```python
from build123d import *

# Parameters (mm, degrees)
CROQUIS1_R              = 2.5
SALIENTE_EXTRUIR1_DEPTH = 6
CROQUIS4_R              = 1
CORTAR_EXTRUIR2_DEPTH   = 3.2


with BuildPart() as part:
    # Croquis1 → Saliente-Extruir1 (new body)
    with BuildSketch(Plane.XY):
        with BuildLine():
            Line((-3.15, -10), (-3.15, -3.545259156))
            Line((-3.15, -3.545259156), (-4, 0))
            ThreePointArc((-4, 0), (0, 4), (4, 0))
            ThreePointArc((4, 0), (2.759247212, -2.590701364), (0.05, -3.545259156))
            Line((0.05, -3.545259156), (0.05, -10))
            Line((0.05, -10), (-3.15, -10))
        make_face()
        Circle(CROQUIS1_R, mode=Mode.SUBTRACT)
    extrude(amount=SALIENTE_EXTRUIR1_DEPTH)

    # Croquis4 → Cortar-Extruir2 (cut)
    with BuildSketch(Plane(origin=(0.05, 0, 0), x_dir=(0, 0, -1), z_dir=(1, 0, 0))):
        with Locations((-3, -6.050719138)):
            Circle(CROQUIS4_R)
    extrude(amount=-CORTAR_EXTRUIR2_DEPTH, mode=Mode.SUBTRACT)


solid = part.part
```
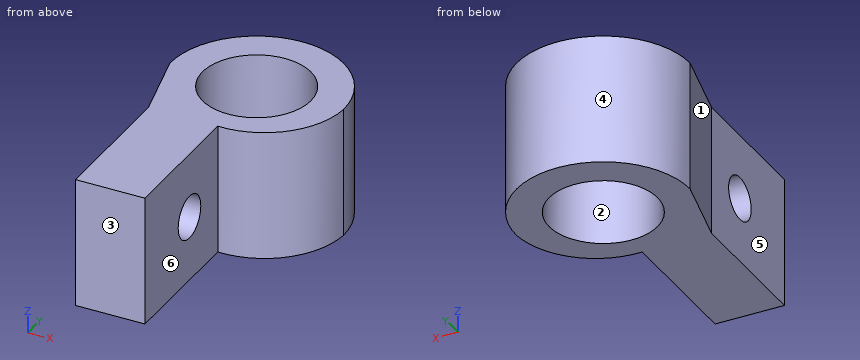
Can you work these out from the model? Positions are in its coordinate system, mm. Face numbers are marked on the shaded views. A direction names the side the tool comes from. Coordinates: 2 decimals unless noted, no trailing zeros. Order: outer loops, then holes, each group sorted by start corner. A loop starts at its lowest first (then second) coordinate and runs counter-clockwise, first axis right, second up. Notation, with made-up numbers: (31.5, 29.25) - (42.5, 29.25) arc R17 ccw to (42.5, 60.25) - close; hole circle Ø5 at (-36, 24.25). An arc over 180 degrees is marked (long way). Answer in a Markdown table with one row per item.
1. For pin 1 (1.5 mm diameter, centred on x = -1, y = -3, fed in from -Z); pin 2 (2 mm diameter, centred on x = -3, z = 1, fed in from +Y); pin 3 (2.5 mm diameter, centred on y = -6.05, z = 3, fed in from +X), each with a flat end and sliding along its axis, tell me the tip position at first contact or that it passes through.
Reply:
| item | result |
|---|---|
| pin 1 | stops at z = 0 |
| pin 2 | stops at y = 3.46 |
| pin 3 | stops at x = 0.05 |
2. Suppose I cut it at D-D (x = 2.25). Please give me the cut outline in (y, z), and give its area (3 significant figures).
Reply:
| item | result |
|---|---|
| outline | (-2.97, 0) - (-1.09, 0) - (-1.09, 6) - (-2.97, 6) - close; (1.09, 0) - (3.31, 0) - (3.31, 6) - (1.09, 6) - close |
| area | 24.6 mm^2 |
3. For the marked faces 4, 5 and 6, which set-ups out of +Z, -Z, +X, -X, +Y, -Y let a thin tool reach every point of the face, with its end or its side?
Reply:
| item | result |
|---|---|
| face 4 | +Z, -Z, +Y |
| face 5 | +Z, -Z, -X, -Y |
| face 6 | +Z, -Z, +X, -Y |
4. If I drill on line 1 along Y through (x, z) = (0, 1.5); line 2 along X through (y, z) = (-6.75, 4.5); line 3 along Y through (x, z) = (-1.4, 3), over which ranges is the centre line in solid material (lowest first)?
Reply:
| item | result |
|---|---|
| line 1 | y = -10 to -2.5, 2.5 to 4 |
| line 2 | x = -3.15 to 0.05 |
| line 3 | y = -10 to -7.05, -5.05 to -2.07, 2.07 to 3.75 |
5. Suppose I cut it at A-A (z = 3). Please give me the cut outline in (x, y), and give its area (3 significant figures).
Reply:
| item | result |
|---|---|
| outline | (-4, 0) - (-3.15, -3.55) - (-3.15, -5.05) - (0.05, -5.05) - (0.05, -3.55) arc R3.75 ccw to (4, 0) arc R4 ccw to start; (-3.15, -10) - (0.05, -10) - (0.05, -7.05) - (-3.15, -7.05) - close; hole circle Ø5 at (0, 0) |
| area | 43.6 mm^2 |
6. Suppose I cut it at C-C (z = 0.6). Please give me the cut outline in (x, y).
Reply:
| item | result |
|---|---|
| outline | (-4, 0) - (-3.15, -3.55) - (-3.15, -10) - (0.05, -10) - (0.05, -3.55) arc R3.75 ccw to (4, 0) arc R4 ccw to start; hole circle Ø5 at (0, 0) |
7. Suppose I cut it at B-B (x = -1). Please give me the cut outline in (y, z).
Reply:
| item | result |
|---|---|
| outline | (-10, 0) - (-2.29, 0) - (-2.29, 6) - (-10, 6) - close; (2.29, 0) - (3.87, 0) - (3.87, 6) - (2.29, 6) - close; hole circle Ø2 at (-6.05, 3) |
8. If we mould it in two halves opening along X, with no side actions, what happens to the marked faces 1, 2 and 3? For each: pulls with the +X half, pulls with the -X half, needs draft (parallel to the pull), parting line crosses it, or undercut.
Reply:
| item | result |
|---|---|
| face 1 | pulls with the -X half |
| face 2 | undercut |
| face 3 | needs draft |
